```python
from build123d import *

# Parameters (mm, degrees)
F0_W     = 114.950902
F0_H     = 131.703299
F1_DEPTH = 25.4
F2_R     = 32.016322
F3_DEPTH = 25.4
F5_DEPTH = 25.4


with BuildPart() as f1:
    # F0 (on Top) → F1 (new body)
    with BuildSketch(Plane.XY):
        with Locations((2.984099, -11.373715)):
            Rectangle(F0_W, F0_H)
    extrude(amount=F1_DEPTH)

    # F2 (on face) → F3 (join)
    with BuildSketch(Plane.XY.offset(25.4)):
        with Locations((5.44278, -5.808717)):
            Circle(F2_R)
    extrude(amount=F3_DEPTH)

    # F4 (on face) → F5 (join)
    with BuildSketch(Plane.XY.offset(50.8)):
        Polygon((13.768743, -3.445501), (10.075767, 3.445501), (2.591765, 5.706847), (-4.299238, 2.013872), (-6.560584, -5.470131), (-2.867608, -12.361133), (4.616394, -14.622479), (11.507397, -10.929504), align=None)
    extrude(amount=F5_DEPTH)


solid = f1.part
```
For this review, take the finished solid that the model builds, in its own axes (mm). A direction names the side the tool comes from. Round coordinates to 2 decimals unless told otherwise and drop trailing zeros. Loops run counter-clockwise (first coordinate to the right, second up) from the corner with the lowest first, then second, coordinate; pieces in that order, holes last.
(1) Wall thickness on line 1 along Z through (x, y) = (-21, -45); line 2 along Z through (x, y) = (-16, -26.5); line 3 along Y through (x, z) = (24.5, 29.5): over which ranges is each line inside the solid? List them lowest first.
Returned:
line 1: z = 0 to 25.4
line 2: z = 0 to 50.8
line 3: y = -31.54 to 19.92
(2) Tool access review of faces 1 (the flat face through (-0.805, 3.886, 63.322)), 2 (the flat face through (6.39, 4.56, 63.32)), 3 (the flat face through (0.822, -13.476, 63.322)): name each direction out of +Z, -Z, +X, -X, +Y, -Y from which nothing blocks a thin tool from reaching the whole face with its end or side.
Returned:
face 1: +Z, -X, +Y
face 2: +Z, +X, +Y
face 3: +Z, -X, -Y
(3) We need section D-D (x = -31.5). Give the boundary of the cut face in (y, z), plus the area to 3 significant figures.
Returned:
outline: (-77.23, 0) - (54.48, 0) - (54.48, 25.4) - (-77.23, 25.4) - close
area: 3,350 mm2
(4) We need section B-B (x = 24.5). Give the boundary of the cut face in (y, z), plus the area to 3 significant figures.
Returned:
outline: (-77.23, 0) - (54.48, 0) - (54.48, 25.4) - (19.92, 25.4) - (19.92, 50.8) - (-31.54, 50.8) - (-31.54, 25.4) - (-77.23, 25.4) - close
area: 4,650 mm2
(5) We need section C-C (y = -62). Give the boundary of the cut face in (x, z), plus the area to 3 significant figures.
Returned:
outline: (-54.49, 0) - (60.46, 0) - (60.46, 25.4) - (-54.49, 25.4) - close
area: 2,920 mm2
(6) Clearance check with flat-ended pins moving along their axes: P1, Ø3, axis at x = 7.5, z = 33.5, coming from the +Y side; P2, Ø4, axis at x = -17, y = 26, coming from the +Z side; P3, Ø10, axis at y = 8, z = 65, coming from the -X side. State where each tip first meets the part, or that it passes through.
Returned:
P1: stops at y = 26.2
P2: stops at z = 25.4
P3: stops at x = -2.46
(7) We need section A-A (z = 66). Give the boundary of the cut face in (x, y), plus the area to 3 significant figures.
Returned:
outline: (-6.56, -5.47) - (-2.87, -12.36) - (4.62, -14.62) - (11.51, -10.93) - (13.77, -3.45) - (10.08, 3.45) - (2.59, 5.71) - (-4.3, 2.01) - close
area: 295 mm2
